Read the model definition and answer for the solid it produces. Units are mm, in the model's axes. A direction names the side the tool comes from. Coordinates: 2 decimals unless noted, no trailing zeros. Order: outer loops, then holes, each group sorted by start corner. A loop starts at its lowest first (then second) coordinate and runs counter-clockwise, first axis right, second up. Notation, with made-up numbers: M 83,60 L 123,60 A16 ccw 123,91 Z; hole C 85,75 d9. An arc over 180 degrees is marked long. Use a Markdown table: item, result. Add a question column.
1) For faces 4 (the face through (-24, 3.175, 0)), 5 (the face through (-18.625, 4.609, -0.141)), 6 (the face through (8, 5, 10)), determine the directions among +Z, -Z, +X, -X, +Y, -Y from which every point of the face is accessible in a straight line to the end or side of a thin tool.
2) Find section B-B on x = 9.95. Write down the section's boundary in (y, z) (3 decimals), plus the area to 3 significant figures.
3) Find section A-A on z = 5. Count the separate pieces of the cut face and the enclosed holes in it, plus the area to 3 significant figures.
4) Each of these flat-tipped pins is pushed along its axis until it touches: pin 1 Ø8 at (x, y) = (16.5, 5.5) entering from -Z; pin 2 Ø1.1 at (y, z) = (6, 3) entering from +X; pin 3 Ø2.5 at (x, z) = (-23, -1) entering from -Y (3 decimals); pin 4 Ø1.5 at (x, z) = (-6, -2) entering from +Y (3 decimals). Where does it stop, or does it pass through?
5) The mould has two halves that part along X. Classify faces 1 (the face through (-27.15, 4.19, 9.19)), 2 (the face through (12.528, 11.147, -0.338)), 3 (the face through (27.033, 4.161, -4.74)): released by +X, released by -X, zero draft, split by the parting line, or undercut.
6) Find the intervals of material crossed by probe 1 along X at (y, z) = (4.25, 5); probe 2 along X at (y, z) = (4.55, -5); probe 3 along Z at (x, y) = (3.5, 5.25), in increasing order. Write a range as [from, to].
7) Find section D-D on y = 12.5. Write down the section's boundary in (x, z).
from build123d import *

# Parameters (mm, degrees)
SKETCH1_W            = 40.1
SKETCH1_H            = 20.1
BOSS_EXTRUDE1_DEPTH  = 3.175
SKETCH2_W            = 2.5
SKETCH2_H            = 20.1
BOSS_EXTRUDE2_DEPTH  = 2
SKETCH3_W            = 20.1
SKETCH3_H            = 2
BOSS_EXTRUDE3_DEPTH  = 8
SKETCH4_R            = 2
CUT_EXTRUDE1_DEPTH   = 30.964739695
FILLET1_R            = 3
FILLET2_R            = 3
FILLET1_OF_MIRROR2_R = 3
FILLET2_OF_MIRROR2_R = 3
SKETCH7_W            = 20
SKETCH7_H            = 20
BOSS_EXTRUDE5_DEPTH  = 6
SKETCH5_R            = 2.6
BOSS_EXTRUDE4_DEPTH  = 5
FILLET4_R            = 3
CHAMFER1_SIZE        = 3
FILLET5_R            = 1


# Some blends are built 0.0001 mm under size
with BuildPart() as part:
    # Sketch1 → Boss-Extrude1 (new body)
    with BuildSketch(Plane(origin=(0, 0, 0), x_dir=(1, 0, 0), z_dir=(0, 1, 0))):
        Rectangle(SKETCH1_W, SKETCH1_H)
    extrude(amount=BOSS_EXTRUDE1_DEPTH)

    # Sketch2 → Boss-Extrude2 (add)
    with BuildSketch(Plane(origin=(0, 3.175, 0), x_dir=(1, 0, 0), z_dir=(0, 1, 0))):
        with Locations((18.8, 0)):
            Rectangle(SKETCH2_W, SKETCH2_H)
    boss_extrude2 = extrude(amount=BOSS_EXTRUDE2_DEPTH)

    # Sketch3 → Boss-Extrude3 (add)
    with BuildSketch(Plane(origin=(20.05, 0, 0), x_dir=(0, 0, -1), z_dir=(1, 0, 0))):
        with Locations((0, 4.175)):
            Rectangle(SKETCH3_W, SKETCH3_H)
    boss_extrude3 = extrude(amount=BOSS_EXTRUDE3_DEPTH)

    # Sketch4 → Cut-Extrude1 (cut, symmetric)
    with BuildSketch(Plane.XZ.offset(-3.175)):
        with Locations(Location((25.05, 5, 0), (0, 0, 270))):
            Circle(SKETCH4_R)
        with Locations(Location((25.05, -5, 0), (0, 0, 270))):
            Circle(SKETCH4_R)
    cut_extrude1 = extrude(amount=CUT_EXTRUDE1_DEPTH, both=True, mode=Mode.SUBTRACT)

    # Fillet1
    # the kernel refuses this fillet: 3 mm, written as the material it takes off along each edge
    with BuildSketch(Plane(origin=(17.55, 5.175, -17.121067812), x_dir=(0, -1, 0), z_dir=(0, 0, 1))) as fillet1_piece_1:
        with BuildLine():
            CenterArc((3, 2.828427125), FILLET1_R, 180, 70.528779366)
            Line((0, 2.828427125), (-0.06, 2.828427125))
            Line((-0.06, 2.828427125), (-0.06, 0))
            Line((-0.06, 0), (0, -0.06))
            ThreePointArc((0, -0.06), (1, -0.06), (1.98, -0.056568542))
            Line((1.98, -0.056568542), (2, 0))
        make_face()
    extrude(amount=34.242135624, mode=Mode.SUBTRACT)

    # Fillet2
    fillet2_edges = [part.edges().sort_by_distance(p)[0] for p in [
        (28.05, 4.175, 10.05),
        (28.05, 4.175, -10.05),
    ]]
    fillet(fillet2_edges, radius=FILLET2_R)

    # Mirror2: Boss-Extrude2, Boss-Extrude3, Cut-Extrude1 across plane
    add(boss_extrude2.mirror(Plane(origin=(0, 0, 0), x_dir=(0, 0, 1), z_dir=(1, 0, 0))))
    add(boss_extrude3.mirror(Plane(origin=(0, 0, 0), x_dir=(0, 0, 1), z_dir=(1, 0, 0))))
    add(cut_extrude1.mirror(Plane(origin=(0, 0, 0), x_dir=(0, 0, 1), z_dir=(1, 0, 0))), mode=Mode.SUBTRACT)

    # Fillet1 of Mirror2
    # the kernel refuses this fillet: 3 mm, written as the material it takes off along each edge
    with BuildSketch(Plane(origin=(-17.55, 5.175, -17.121067812), x_dir=(-1, 0, 0), z_dir=(0, 0, 1))) as fillet1_of_mirror2_piece_1:
        with BuildLine():
            CenterArc((2.828427125, 3), FILLET1_OF_MIRROR2_R, 199.471220634, 70.528779366)
            Line((0, 2), (-0.056568542, 1.98))
            ThreePointArc((-0.056568542, 1.98), (-0.06, 1), (-0.06, 0))
            Line((-0.06, 0), (0, -0.06))
            Line((0, -0.06), (2.828427125, -0.06))
            Line((2.828427125, -0.06), (2.828427125, 0))
        make_face()
    extrude(amount=34.242135624, mode=Mode.SUBTRACT)

    # Fillet2 of Mirror2
    fillet2_of_mirror2_edges = [part.edges().sort_by_distance(p)[0] for p in [
        (-28.05, 4.175, 10.05),
        (-28.05, 4.175, -10.05),
    ]]
    fillet(fillet2_of_mirror2_edges, radius=FILLET2_OF_MIRROR2_R)

    # Sketch7 → Boss-Extrude5 (add)
    with BuildSketch(Plane(origin=(0, 3.175, 0), x_dir=(1, 0, 0), z_dir=(0, 1, 0))):
        with Locations((9.95, 0)):
            Rectangle(SKETCH7_W, SKETCH7_H)
    extrude(amount=BOSS_EXTRUDE5_DEPTH)

    # Sketch5 → Boss-Extrude4 (add)
    with BuildSketch(Plane(origin=(0, 9.175, 0), x_dir=(1, 0, 0), z_dir=(0, 1, 0))):
        with Locations(Location((9.95, 0, 0), (0, 0, 270))):
            Circle(SKETCH5_R)
    extrude(amount=BOSS_EXTRUDE4_DEPTH)

    # Fillet4
    fillet4_edges = [part.edges().sort_by_distance(p)[0] for p in [
        (-0.05, 3.175, 0),
    ]]
    fillet(fillet4_edges, radius=FILLET4_R)

    # Chamfer1
    chamfer1_edges = [part.edges().sort_by_distance(p)[0] for p in [
        (19.95, 9.175, 0),
        (9.95, 9.175, -10),
        (-0.05, 9.175, 0),
        (9.95, 9.175, 10),
    ]]
    chamfer(chamfer1_edges, length=CHAMFER1_SIZE - 0.0001)  # a hair under: the kernel refuses the full size

    # Fillet5
    fillet5_edges = [part.edges().sort_by_distance(p)[0] for p in [
        (9.95, 14.175, -2.6),
    ]]
    fillet(fillet5_edges, radius=FILLET5_R)


solid = part.part
Check result:
| question | item | result |
|---|---|---|
| 1 | face 4 | +Z, -Z, -X, -Y |
| 1 | face 5 | +Z, -Z, +Y |
| 1 | face 6 | +Z, +Y |
| 2 | outline | M 0,-10.05 L 3.175,-10.05 L 3.175,-10 L 6.175,-10 L 9.175,-7 L 9.175,-2.6 L 13.175,-2.6 A1 ccw 14.175,-1.6 L 14.175,1.6 A1 ccw 13.175,2.6 L 9.175,2.6 L 9.175,7 L 6.175,10 L 3.175,10 L 3.175,10.05 L 0,10.05 Z |
| 2 | area | 200 mm2 |
| 3 | separate pieces | 3 |
| 3 | enclosed holes | 0 |
| 3 | area | 260 mm2 |
| 4 | pin 1 | stops at z = -10.05 |
| 4 | pin 2 | stops at x = 19.95 |
| 4 | pin 3 | stops at y = 3.175 |
| 4 | pin 4 | stops at y = 3.175 |
| 5 | face 1 | released by -X |
| 5 | face 2 | split by the parting line |
| 5 | face 3 | undercut |
| 6 | probe 1 | x = [-28.05, -27.05], [-23.05, -18.21], [-0.75, 23.05], [27.05, 28.05] |
| 6 | probe 2 | x = [-28.05, -27.05], [-23.05, -18.55], [-0.53, 23.05], [27.05, 28.05] |
| 6 | probe 3 | z = [-10, 10] |
| 7 | outline | C 9.95,0 d5.2 |
